Build history of the part. All positions in model axes, mm. Face numbers are marked on the shaded views. Round coordinates to 2 decimals unless told otherwise and drop trailing zeros. Loops run counter-clockwise (first coordinate to the right, second up) from the corner with the lowest first, then second, coordinate; pieces in that order, holes last.
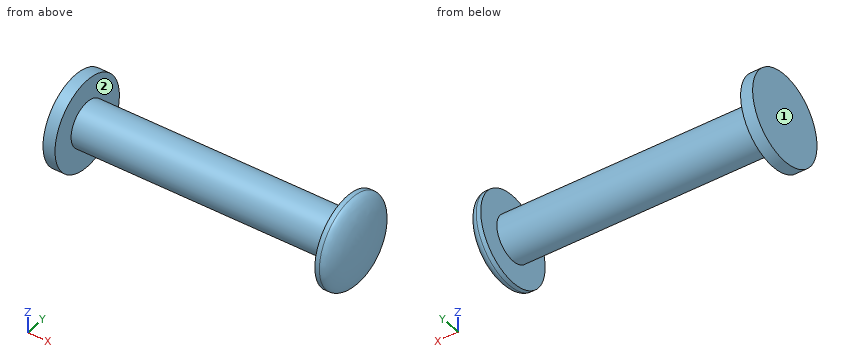
from build123d import *

# Parameters (mm, degrees)
CROQUIS1_R              = 3
SALIENTE_EXTRUIR1_DEPTH = 0.8
CROQUIS2_R              = 1.5
SALIENTE_EXTRUIR2_DEPTH = 17.3
CROQUIS3_R              = 3
SALIENTE_EXTRUIR3_DEPTH = 0.3
C_PULA1_FACE_RADIUS     = 3
C_PULA1_HEIGHT          = 1


with BuildPart() as part:
    # Croquis1 → Saliente-Extruir1 (new body)
    with BuildSketch(Plane(origin=(0, 0, 0), x_dir=(0, 0, -1), z_dir=(1, 0, 0))):
        Circle(CROQUIS1_R)
    extrude(amount=SALIENTE_EXTRUIR1_DEPTH)

    # Croquis2 → Saliente-Extruir2 (add)
    with BuildSketch(Plane(origin=(0.8, 0, 0), x_dir=(0, 0, -1), z_dir=(1, 0, 0))):
        Circle(CROQUIS2_R)
    extrude(amount=SALIENTE_EXTRUIR2_DEPTH)

    # Croquis3 → Saliente-Extruir3 (add)
    with BuildSketch(Plane(origin=(18.1, 0, 0), x_dir=(0, 0, -1), z_dir=(1, 0, 0))):
        Circle(CROQUIS3_R)
    extrude(amount=SALIENTE_EXTRUIR3_DEPTH)

    # Cúpula1: an elliptical dome of height H over a round flat face of radius A is half a spheroid: the quarter ellipse of half axes A and H revolved about the face's axis
    with BuildSketch(Plane((18.4, 0, 0), x_dir=(0, 0, 1), z_dir=(0, 1, 0)), mode=Mode.PRIVATE) as c_pula1_quarter:
        Ellipse(C_PULA1_FACE_RADIUS, C_PULA1_HEIGHT)
        Rectangle(C_PULA1_FACE_RADIUS, C_PULA1_HEIGHT, align=(Align.MIN, Align.MIN), mode=Mode.INTERSECT)
    revolve(c_pula1_quarter.sketch, axis=Axis((18.4, 0, 0), (1, 0, 0)))


solid = part.part
(1) Pin check, flat tips, straight feed: P1, Ø1, axis at y = 1, z = 0.5, coming from the +X side; P2, Ø2, axis at x = 8, y = 1.5, coming from the +Z side; P3, Ø2, axis at x = 3, y = -1, coming from the -Z side. Stop position of each tip, or through.
Responses:
P1: stops at x = 19.38
P2: stops at z = 1.41
P3: stops at z = -1.5
(2) Pull direction X, two halves, no side cores. Call the marked faces 1 and 2: +X half, -X half, draft (parallel to the pull), parting line (faces both ways), or undercut.
Responses:
face 1: -X half
face 2: undercut
(3) Slice it at A-A on x = 7.25. List the corners of the cut face in (y, z).
Responses:
outline: circle Ø3 at (0, 0)
(4) Probe line 1 (X direction, y = 2.25, z = 0.5); line 2 (X direction, y = -1.5, z = -2.5); line 3 (Y direction, x = 2.5, z = 1.25). List the from-to ranges inside material, lowest first.
Responses:
line 1: x = 0 to 0.8, 18.1 to 19.04
line 2: x = 0 to 0.8, 18.1 to 18.64
line 3: y = -0.83 to 0.83
